Source: three-view drawing plus pictorial views. Frame: mm from the lowest corner of the part. A direction names the side the tool comes from. Round coordinates to 2 decimals unless told otherwise and drop trailing zeros. Write each loop counter-clockwise with the first axis right and the second up, starting at its lowest first coordinate (ties: lowest second). Pieces come first, ordered by that corner, then holes. Notation, with made-up numbers: M 59,77.5 L 106,77.5 A24 cw 106,112.5 Z; hole C 5.5,49.25 d4. An arc over 180 degrees is marked long. Answer in a Markdown table with one row per item.
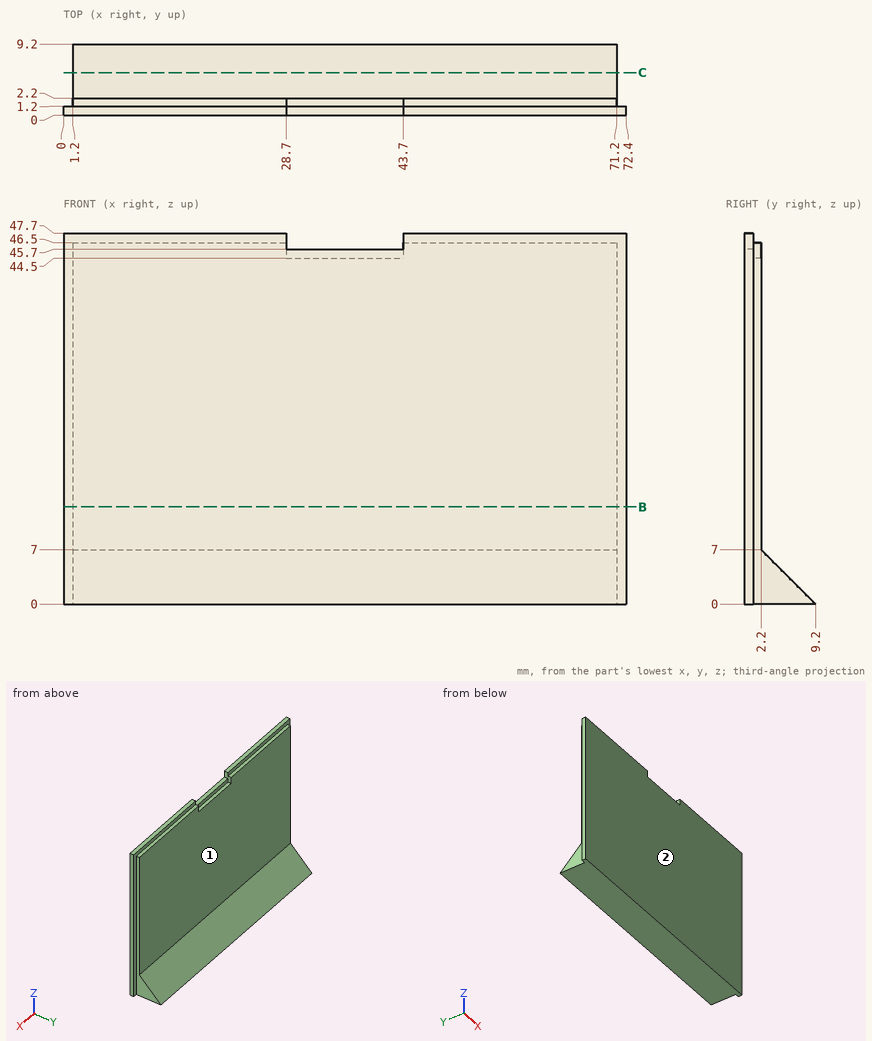
Q1. Material intervals for probe 1 along Z at (x, y) = (54, 1.75); probe 2 along Y at (x, z) = (64, 40.5); probe 3 along Z at (x, y) = (59.5, 8), sorted ascending.
Solutions:
| item | result |
|---|---|
| probe 1 | z = 0 to 46.5 |
| probe 2 | y = 0 to 2.2 |
| probe 3 | z = 0 to 1.2 |
Q2. Section B-B (z = 12.5). Return loops of the section in (x, y).
Solutions:
| item | result |
|---|---|
| outline | M 0,0 L 72.4,0 L 72.4,1.2 L 71.2,1.2 L 71.2,2.2 L 1.2,2.2 L 1.2,1.2 L 0,1.2 Z |
Q3. Access query for the marked faces 1 and 2. Directions: +Z, -Z, +X, -X, +Y, -Y. A direction counts if a zero-diameter tool reaches every point of the face in a straight line with its end or side. Return the directions, or none.
Solutions:
| item | result |
|---|---|
| face 1 | +Z, +X, -X, +Y |
| face 2 | +Z, -Z, +X, -X, -Y |
Q4. Section C-C (y = 5.5). Return loops of the section in (x, z), and give its area (3 significant figures).
Solutions:
| item | result |
|---|---|
| outline | M 1.2,0 L 71.2,0 L 71.2,3.7 L 1.2,3.7 Z |
| area | 259 mm2 |
Q5. Contact query for flat-ended pins moving along their axis: pin 1 Ø23 at (x, z) = (11.5, 20.5) entering from +Y; pin 2 Ø0.6 at (x, y) = (34, 0.5) entering from +Z; pin 3 Ø4 at (y, z) = (4.5, 34) entering from -X. Output: stop coordinate, or through.
Solutions:
| item | result |
|---|---|
| pin 1 | stops at y = 2.2 |
| pin 2 | stops at z = 45.7 |
| pin 3 | passes through |
